Work out the finished part from the listing and answer in its coordinate system (mm). Round coordinates to 2 decimals unless told otherwise and drop trailing zeros. Loops run counter-clockwise (first coordinate to the right, second up) from the corner with the lowest first, then second, coordinate; pieces in that order, holes last. Notation, with made-up numbers: (53, 89) - (90, 89) arc R16 cw to (90, 100) - close; hole circle Ø9 at (60, 68). An arc over 180 degrees is marked (long way). Answer as CSV lines item,"result". Start each with the question number.
Q1. Straight lines are drawn through the part: L1, parallel to X at y = 9, z = -179; L2, parallel to Y at x = -626.5, z = -813; L3, parallel to Z at x = 495, y = 14. For each, find the intervals that lie inside material, in ascending order. Write a range as [from, to].
Q2. Section A-A on y = 15 is taken. Write down the section's boundary in (x, z).
Q3. Each of these flat-tipped pins is pushed along its axis until it touches: pin 1 Ø6 at (x, y) = (232, 13.5) entering from +Z; pin 2 Ø10 at (x, y) = (470, 24.5) entering from -Z. Where does it stop, or does it pass through?
Q4. Section B-B on z = -179 is taken. Write down the section's boundary in (x, y), then the cut area to 3 significant figures.
Q5. Section C-C on x = 787.5 is taken. Write down the section's boundary in (y, z).
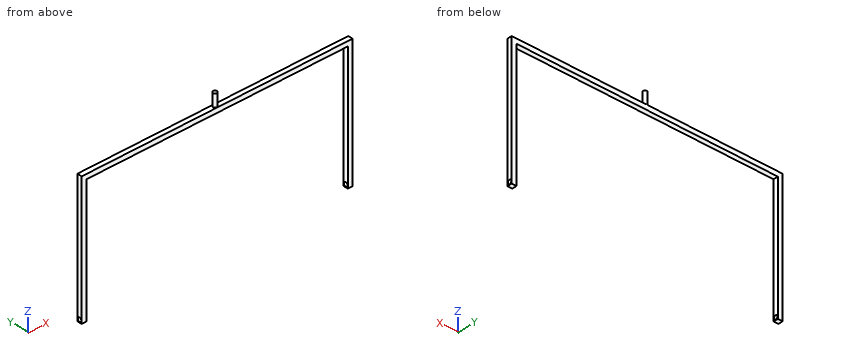
```python
from build123d import *

# Parameters (mm, degrees)
EXTRUDE_1_DEPTH     = 30
SKETCH_3_R          = 12.5
CUT_EXTRUDE_1_DEPTH = 1903.825267858
SKETCH_5_R          = 12.5
CUT_EXTRUDE_2_DEPTH = 1355.510981868
EXTRUDE_START       = -110
SKETCH_7_R          = 12.5
EXTRUDE_3_DEPTH     = 110


with BuildPart() as part:
    # Эскиз1 → Бобышка-Вытянуть1 (new body)
    with BuildSketch(Plane(origin=(0, 0, 0), x_dir=(1, 0, 0), z_dir=(0, 1, 0))):
        Polygon((1070, 0), (-642, 0), (-642, 830), (-612, 830), (-612, 30), (1040, 30), (1040, 830), (1070, 830), align=None)
    extrude(amount=EXTRUDE_1_DEPTH)

    # Эскиз3 → Вырез-Вытянуть1 (cut, through all)
    with BuildSketch(Plane.ZY.offset(642)):
        with Locations((-813, 15)):
            Circle(SKETCH_3_R)
    extrude(amount=-CUT_EXTRUDE_1_DEPTH, mode=Mode.SUBTRACT)

    # Эскиз5 → Вырез-Вытянуть2 (cut, through all)
    with BuildSketch(Plane.XY):
        with Locations((214, 15)):
            Circle(SKETCH_5_R)
    extrude(amount=-CUT_EXTRUDE_2_DEPTH, mode=Mode.SUBTRACT)

    # Эскиз7 → Бобышка-Вытянуть3 (add)
    with BuildSketch(Plane(origin=(0, 0, -30), x_dir=(-1, 0, 0), z_dir=(0, 0, -1)).offset(EXTRUDE_START)):
        with Locations((-214, 15)):
            Circle(SKETCH_7_R)
    extrude(amount=EXTRUDE_3_DEPTH)


solid = part.part
```
Findings:
1,L1,"x = [-642, -612], [1040, 1070]"
1,L2,"y = [0, 2.5], [27.5, 30]"
1,L3,"z = [-30, 0]"
2,outline,"(-642, -830) - (-612, -830) - (-612, -825.5) - (-642, -825.5) - close; (-642, -800.5) - (-612, -800.5) - (-612, -30) - (1040, -30) - (1040, -800.5) - (1070, -800.5) - (1070, 0) - (226.5, 0) - (226.5, 80) - (201.5, 80) - (201.5, 0) - (-642, 0) - close; (1040, -830) - (1070, -830) - (1070, -825.5) - (1040, -825.5) - close"
3,pin 1,"stops at z = 0"
3,pin 2,"stops at z = -30"
4,outline,"(-642, 0) - (-612, 0) - (-612, 30) - (-642, 30) - close; (1040, 0) - (1070, 0) - (1070, 30) - (1040, 30) - close"
4,area,"1,800 mm^2"
5,outline,"(0, -30) - (30, -30) - (30, 0) - (0, 0) - close"
